Geometry check sheet. Reference: drawing and pictorial views, mm from the part's lowest x, y, z. Round coordinates to 2 decimals unless told otherwise and drop trailing zeros. Order: outer loops, then holes, each group sorted by start corner. A loop starts at its lowest first (then second) coordinate and runs counter-clockwise, first axis right, second up. Notation, with made-up numbers: (29.5, 66.25) -> (65.5, 66.25) arc R22 cw to (65.5, 76.25) -> close; hole circle Ø5 at (18.25, 53.5). An arc over 180 degrees is marked (long way). Return JSON: item names as keys, results as strings. Group by question number.
1) Depth check by flat-ended pin: pin 1 (2.5 mm diameter, centred on x = 200.5, z = 1.5, fed in from +Y); pin 2 (2.5 mm diameter, centred on x = 16, z = 2.5, fed in from -Y); pin 3 (2.5 mm diameter, centred on y = 38, z = 2, fed in from -X). Enter the tip coordinate at first touch or a pass-through.
2) Section check A-A on z = 1.2. Enter the section's corners in (x, y).
3) Scan lines: L1, parallel to Y at x = 71, z = 1.35; L2, parallel to X at y = 35.5, z = 3.3. Record each from-to range of solid material in increasing order.
4) Section check C-C on y = 14.5. Enter the section's corners in (x, z), plus the area to 3 significant figures.
5) Section check B-B on x = 178. Enter the section's corners in (y, z), plus the area to 3 significant figures.
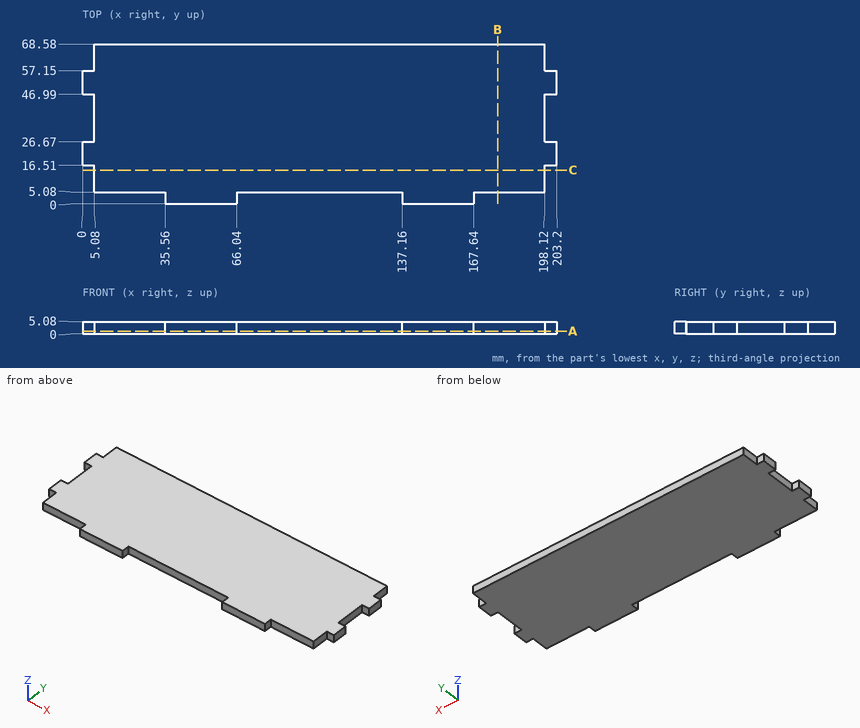
Check result:
{
 "1": {"pin 1": "y = 57.15", "pin 2": "y = 5.08", "pin 3": "x = 5.08"},
 "2": {"outline": "(0, 16.51) -> (5.08, 16.51) -> (5.08, 5.08) -> (35.56, 5.08) -> (35.56, 0) -> (66.04, 0) -> (66.04, 5.08) -> (137.16, 5.08) -> (137.16, 0) -> (167.64, 0) -> (167.64, 5.08) -> (198.12, 5.08) -> (198.12, 16.51) -> (203.2, 16.51) -> (203.2, 26.67) -> (198.12, 26.67) -> (198.12, 46.99) -> (203.2, 46.99) -> (203.2, 57.15) -> (198.12, 57.15) -> (198.12, 68.58) -> (5.08, 68.58) -> (5.08, 57.15) -> (0, 57.15) -> (0, 46.99) -> (5.08, 46.99) -> (5.08, 26.67) -> (0, 26.67) -> close"},
 "3": {"L1": "5.08 to 68.58", "L2": "5.08 to 198.12"},
 "4": {"outline": "(5.08, 0) -> (198.12, 0) -> (198.12, 5.08) -> (5.08, 5.08) -> close", "area": "981 mm^2"},
 "5": {"outline": "(5.08, 0) -> (68.58, 0) -> (68.58, 5.08) -> (5.08, 5.08) -> close", "area": "323 mm^2"}
}
